Geometry check sheet. Reference: the model listing, model coordinates, mm. Face numbers are marked on the shaded views. Give positions to 0.01 mm unless a question says otherwise; leave off trailing zeros. Write each loop counter-clockwise with the first axis right and the second up, starting at its lowest first coordinate (ties: lowest second). Pieces come first, ordered by that corner, then holes. Notation, with made-up numbers: (15, 79) - (41, 79) arc R22 cw to (41, 118) - close; hole circle Ø2 at (67, 81). An arc over 180 degrees is marked (long way). Use a Markdown table: item, result.
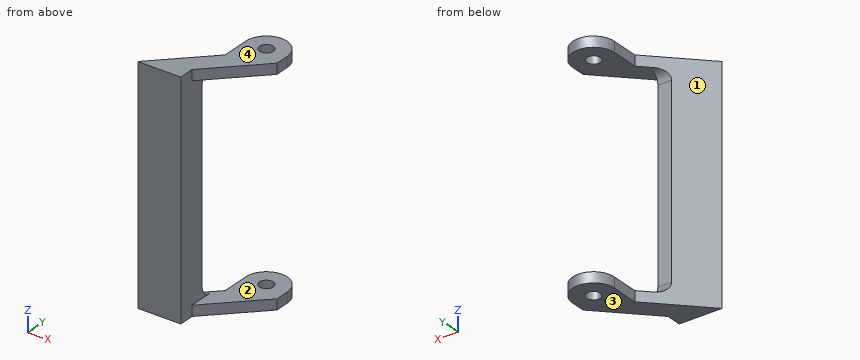
```python
from build123d import *

# Parameters (mm, degrees)
EXTRUDE1_DEPTH = 3
EXTRUDE2_DEPTH = 66
EXTRUDE3_START = -3
EXTRUDE3_DEPTH = 3
SKETCH2_R      = 2
EXTRUDE4_DEPTH = 3
EXTRUDE5_START = -3
SKETCH6_R      = 2
EXTRUDE5_DEPTH = 3
FILLET3_R      = 3


with BuildPart() as part:
    # Sketch1 → Extrude1 (new body)
    with BuildSketch(Plane.XY):
        with BuildLine():
            Line((-8.805401881, -5.201299994), (-2.663266257, 0.94083563))
            Line((-2.663266257, 0.94083563), (-2.663266257, 8.94083563))
            ThreePointArc((-2.663266257, 8.94083563), (3.336733743, 14.94083563), (9.336733743, 8.94083563))
            Line((9.336733743, 8.94083563), (9.336733743, 4.94083563))
            Line((9.336733743, 4.94083563), (-4.805401881, -9.201299994))
            Line((-4.805401881, -9.201299994), (-4.805401881, -5.201299994))
            Line((-4.805401881, -5.201299994), (-8.805401881, -5.201299994))
        make_face()
    extrude(amount=EXTRUDE1_DEPTH)

    # Sketch3 → Extrude2 (add)
    with BuildSketch(Plane.XY):
        Polygon((-8.805401881, -5.201299994), (-4.805401881, -5.201299994), (-4.805401881, -13.601299994), (-17.205401881, -13.601299994), align=None)
    extrude(amount=EXTRUDE2_DEPTH)

    # Sketch4 → Extrude3 (add)
    with BuildSketch(Plane.XY.offset(66).offset(EXTRUDE3_START)):
        with BuildLine():
            Line((-8.805401881, -5.201299994), (-4.805401881, -5.201299994))
            Line((-4.805401881, -5.201299994), (-4.805401881, -9.201299994))
            Line((-4.805401881, -9.201299994), (9.336733743, 4.94083563))
            Line((9.336733743, 4.94083563), (9.336733743, 8.94083563))
            ThreePointArc((9.336733743, 8.94083563), (3.336733743, 14.94083563), (-2.663266257, 8.94083563))
            Line((-2.663266257, 8.94083563), (-2.663266257, 0.94083563))
            Line((-2.663266257, 0.94083563), (-8.805401881, -5.201299994))
        make_face()
    extrude(amount=EXTRUDE3_DEPTH)

    # Sketch2 → Extrude4 (cut)
    with BuildSketch(Plane.XY.offset(3)):
        with Locations((3.336733743, 8.94083563)):
            Circle(SKETCH2_R)
    extrude(amount=-EXTRUDE4_DEPTH, mode=Mode.SUBTRACT)

    # Sketch6 → Extrude5 (cut)
    with BuildSketch(Plane(origin=(0, 0, 63), x_dir=(-1, 0, 0), z_dir=(0, 0, -1)).offset(EXTRUDE5_START)):
        with Locations(Location((-3.336733743, 8.94083563, 0), (0, 0, 180))):
            Circle(SKETCH6_R)
    extrude(amount=EXTRUDE5_DEPTH, mode=Mode.SUBTRACT)

    # Fillet3
    fillet3_edges = [part.edges().sort_by_distance(p)[0] for p in [
        (-6.805401881, -5.201299994, 3),
        (-6.805401881, -5.201299994, 63),
    ]]
    fillet(fillet3_edges, radius=FILLET3_R)


solid = part.part
```
1) Depth check by flat-ended pin: P1, Ø9, axis at y = -7, z = 28.5, coming from the +X side; P2, Ø8, axis at y = -3.5, z = 52, coming from the -X side; P3, Ø3.5, axis at y = 6, z = 64.5, coming from the -X side. Enter the tip coordinate at first touch or a pass-through.
Working result:
| item | result |
|---|---|
| P1 | stops at x = -4.81 |
| P2 | stops at x = -11.1 |
| P3 | stops at x = -2.66 |
2) Section check A-A on x = 6.5. Record the boundary of the cut face in (y, z), then the cut area to 3 significant figures.
Working result:
| item | result |
|---|---|
| outline | (2.1, 0) - (14.04, 0) - (14.04, 3) - (2.1, 3) - close; (2.1, 63) - (14.04, 63) - (14.04, 66) - (2.1, 66) - close |
| area | 71.6 mm² |
3) Section check D-D on y = -12. Record the boundary of the cut face in (x, z), then the cut area to 3 significant figures.
Working result:
| item | result |
|---|---|
| outline | (-15.6, 0) - (-4.81, 0) - (-4.81, 66) - (-15.6, 66) - close |
| area | 713 mm² |
4) Material ranges on L1, parallel to Z at x = -2, y = -1.5; L2, parallel to Y at x = -6.25, z = 29; L3, parallel to X at y = -8, z = 46, recorded low to high. Write a range as from..to.
Working result:
| item | result |
|---|---|
| L1 | z = 0..3, 63..66 |
| L2 | y = -13.6..-5.2 |
| L3 | x = -11.6..-4.81 |
5) Section check C-C on z = 4. Record the boundary of the cut face in (x, y).
Working result:
| item | result |
|---|---|
| outline | (-17.21, -13.6) - (-4.81, -13.6) - (-4.81, -4.44) - (-8.04, -4.44) - close |
6) Mould release check, pull along Z, two halves, no side actions. Record for the marked faces 1, 2, 3 and 4: pulls with the +Z half, pulls with the -Z half, needs draft (parallel to the pull), parting line crosses it, or undercut.
Working result:
| item | result |
|---|---|
| face 1 | needs draft |
| face 2 | undercut |
| face 3 | pulls with the -Z half |
| face 4 | pulls with the +Z half |
7) Section check B-B on x = -6.5. Record the boundary of the cut face in (y, z).
Working result:
| item | result |
|---|---|
| outline | (-13.6, 0) - (-2.9, 0) - (-2.9, 3.08) arc R3 cw to (-5.2, 6) - (-5.2, 60) arc R3 cw to (-2.9, 62.92) - (-2.9, 66) - (-13.6, 66) - close |
